Source: CAD feature listing. Evaluate the final solid. Frame: model axes, mm. A direction names the side the tool comes from. Round coordinates to 2 decimals unless told otherwise and drop trailing zeros. Order: outer loops, then holes, each group sorted by start corner. A loop starts at its lowest first (then second) coordinate and runs counter-clockwise, first axis right, second up. Notation, with made-up numbers: M 41.5,30.25 L 49.5,30.25 A14 ccw 49.5,40.25 Z; hole C 76.5,-25 d6. An arc over 180 degrees is marked long. Answer in a Markdown table with one row per item. Add a question column.
```python
from build123d import *

# Parameters (mm, degrees)
SKETCH1_W                = 124
SKETCH1_H                = 184
SKETCH1_W_2              = 120
SKETCH1_H_2              = 180
BOSS_EXTRUDE1_DEPTH      = 4
SKETCH1_3_W              = 120
SKETCH1_3_H              = 180
BOSS_EXTRUDE2_DEPTH      = 30
BOSS_EXTRUDE2_DEPTH_BACK = 40


with BuildPart() as part:
    # Sketch1 → Boss-Extrude1 (new body)
    with BuildSketch(Plane(origin=(0, 0, 0), x_dir=(1, 0, 0), z_dir=(0, 1, 0))):
        with Locations((0, -0.402295225)):
            Rectangle(SKETCH1_W, SKETCH1_H)
        with Locations((0, -0.402295225)):
            Rectangle(SKETCH1_W_2, SKETCH1_H_2, mode=Mode.SUBTRACT)
    extrude(amount=BOSS_EXTRUDE1_DEPTH)

    # Sketch1_3 → Boss-Extrude2 (add, two sides)
    with BuildSketch(Plane(origin=(0, 0, 0), x_dir=(1, 0, 0), z_dir=(0, 1, 0))) as boss_extrude2_sk:
        with Locations((0, -0.402295225)):
            Rectangle(SKETCH1_3_W, SKETCH1_3_H)
    extrude(amount=BOSS_EXTRUDE2_DEPTH)
    extrude(boss_extrude2_sk.sketch, amount=-BOSS_EXTRUDE2_DEPTH_BACK)


solid = part.part
```
(1) Cut plane C-C (y = -29). Return loops of the section in (x, z), and give its area (3 significant figures).
(2) Cut plane B-B (x = -7.5). Return loops of the section in (y, z), and give its area (3 significant figures).
(3) Pin query (flat end, axial travel): pin 1 (10 mm diameter, centred on x = 13, y = -27, fed in from -Z); pin 2 (10 mm diameter, centred on y = -26, z = 7.5, fed in from -X); pin 3 (13 mm diameter, centred on x = 8.5, y = 22.5, fed in from +Z). Return the tip coordinate at first contact, or that it passes through.
(4) Access query for faces 1 (the face through (-60, -20, 2)), 2 (the face through (-1, 17, 90.402)), 3 (the face through (-1, -20, -89.598)). Directions: +Z, -Z, +X, -X, +Y, -Y. A direction counts if a zero-diameter tool reaches every point of the face in a straight line with its end or side. Return the directions, or none.
(5) Cut plane A-A (z = -38). Return loops of the section in (x, y), and give its area (3 significant figures).
(6) Line query: line 1 (Z direction, x = -24.5, y = -22.5); line 2 (X direction, y = -37, z = 73.5). Output: solid intervals per line, ascending. Write a range as from..to.
Answer list:
| question | item | result |
|---|---|---|
| 1 | outline | M -60,-89.6 L 60,-89.6 L 60,90.4 L -60,90.4 Z |
| 1 | area | 21,600 mm² |
| 2 | outline | M -40,-89.6 L 0,-89.6 L 0,-91.6 L 4,-91.6 L 4,-89.6 L 30,-89.6 L 30,90.4 L 4,90.4 L 4,92.4 L 0,92.4 L 0,90.4 L -40,90.4 Z |
| 2 | area | 12,600 mm² |
| 3 | pin 1 | z = -89.6 |
| 3 | pin 2 | x = -60 |
| 3 | pin 3 | z = 90.4 |
| 4 | face 1 | +Z, -Z, -X, -Y |
| 4 | face 2 | +Z, +X, -X, +Y |
| 4 | face 3 | -Z, +X, -X, -Y |
| 5 | outline | M -62,0 L -60,0 L -60,-40 L 60,-40 L 60,0 L 62,0 L 62,4 L 60,4 L 60,30 L -60,30 L -60,4 L -62,4 Z |
| 5 | area | 8,420 mm² |
| 6 | line 1 | -89.6..90.4 |
| 6 | line 2 | -60..60 |
